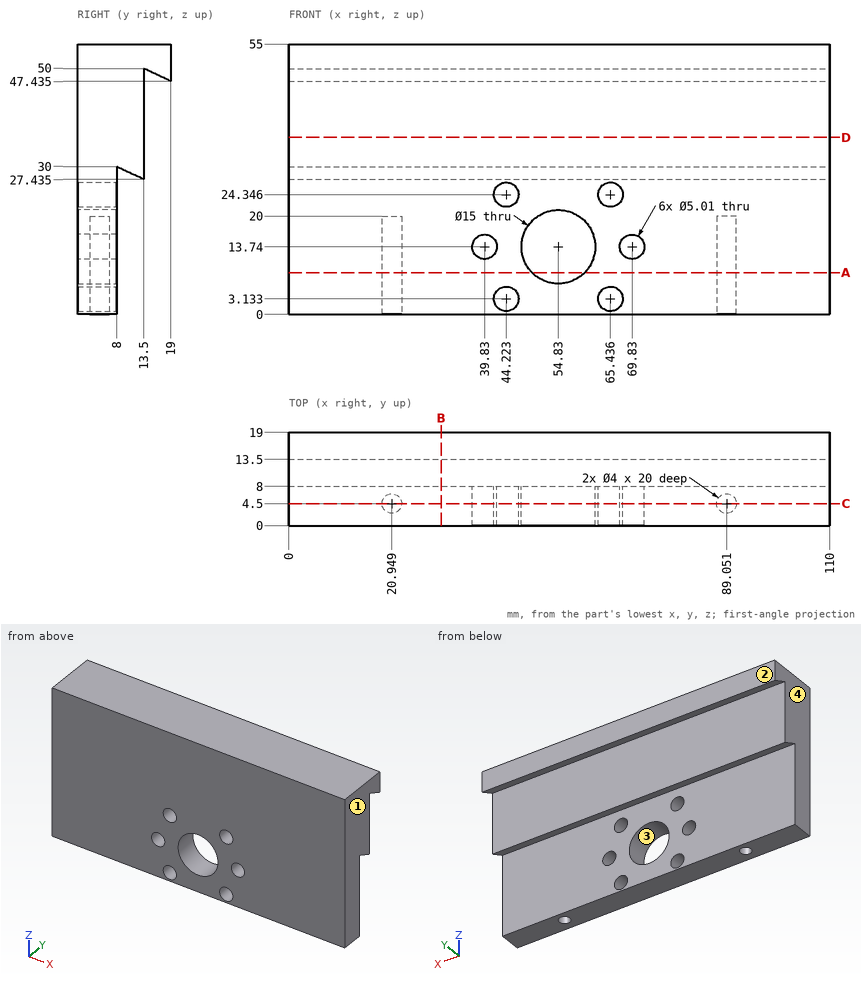
Verification items for this drawing (mm, ordinates from the low corner). Give positions to 0.01 mm unless a question says otherwise; leave off trailing zeros. Loops run counter-clockwise (first coordinate to the right, second up) from the corner with the lowest first, then second, coordinate; pieces in that order, holes last. Notation, with made-up numbers: M 75,56 L 103,56 A12 ccw 103,71 Z; hole C 40.5,63.5 d10. An arc over 180 degrees is marked long. Answer as a JSON object with one key per item and string values. Group by question number.
Item 1: Sectioned sample at B-B on x = 31. Record the boundary of the cut face in (y, z) (1 decimal).
Item 2: Sectioned sample at D-D on z = 36. Record the boundary of the cut face in (x, y), plus the area to 4 significant figures.
Item 3: Sectioned sample at A-A on z = 8.5. Record the boundary of the cut face in (x, y) (1 decimal).
Item 4: Mould release check, pull along X, two halves, no side actions. Record for the marked faces 1, 2, 3 and 4: pulls with the +X half, pulls with the -X half, needs draft (parallel to the pull), parting line crosses it, or undercut.
Item 5: Sectioned sample at C-C on y = 4.5. Record the boundary of the cut face in (x, z) (1 decimal), plus the area to 4 significant figures.
Item 6: Material ranges on L1, parallel to Y at x = 89, z = 18; L2, parallel to Z at x = 43.5, y = 4 (1 decimal); L3, parallel to Y at x = 36, z = 21, recorded low to high.
Item 7: Gauge pin test, flat ends, axial feed: pin 1 (4 mm diameter, centred on x = 16.5, y = 13, fed in from -Z) (1 decimal); pin 2 (3.5 mm diameter, centred on x = 89.05, y = 4.5, fed in from -Z); pin 3 (11.5 mm diameter, centred on x = 55.5, z = 34.5, fed in from +Y). Record the tip position at first contact, or that the pin passes through.
Findings below:
{
 "1": {"outline": "M 0,0 L 8,0 L 8,30 L 13.5,27.4 L 13.5,50 L 19,47.4 L 19,55 L 0,55 Z"},
 "2": {"outline": "M 0,0 L 110,0 L 110,13.5 L 0,13.5 Z", "area": "1,485 mm2"},
 "3": {"outline": "M 0,0 L 49.5,0 L 49.5,8 L 0,8 Z; M 60.2,0 L 110,0 L 110,8 L 60.2,8 Z; hole C 20.9,4.5 d4; hole C 89.1,4.5 d4"},
 "4": {"face 1": "pulls with the +X half", "face 2": "needs draft", "face 3": "undercut", "face 4": "pulls with the -X half"},
 "5": {"outline": "M 0,0 L 18.9,0 L 18.9,20 L 22.9,20 L 22.9,0 L 87.1,0 L 87.1,20 L 91.1,20 L 91.1,0 L 110,0 L 110,55 L 0,55 Z; hole C 39.8,13.7 d5; hole C 44.2,3.1 d5; hole C 44.2,24.3 d5; hole C 54.8,13.7 d15; hole C 65.4,3.1 d5; hole C 65.4,24.3 d5; hole C 69.8,13.7 d5", "area": "5,595 mm2"},
 "6": {"L1": "0 to 2.5, 6.5 to 8", "L2": "0 to 0.7, 5.5 to 21.9, 26.7 to 55", "L3": "0 to 8"},
 "7": {"pin 1": "z = 27.4", "pin 2": "z = 20", "pin 3": "y = 13.5"}
}
